Verification items for this drawing (mm, ordinates from the low corner). A direction names the side the tool comes from. Round coordinates to 2 decimals unless told otherwise and drop trailing zeros. Write each loop counter-clockwise with the first axis right and the second up, starting at its lowest first coordinate (ties: lowest second). Pieces come first, ordered by that corner, then holes. Notation, with made-up numbers: M -35,73.5 L -2,73.5 A21 ccw -2,91.5 Z; hole C 62,-39 d1. An arc over 180 degrees is marked long. One line per question, with ' | ' between items. Start each with the question number.
Q1. Tool access check on the marked faces 4 and 5. Record the directions out of +Z, -Z, +X, -X, +Y, -Y that give a thin tool (end or side, any length) a straight path to the whole face; none if there is none.
Q2. Cross-section at B-B (y = 8). Record the boundary of the cut face in (x, z).
Q3. Thickness scan on line 1 along Z through (x, y) = (18, 20.5); line 2 along Y through (x, z) = (35.5, 3.25); line 3 along Y through (x, z) = (34, 24.75). Record the ranges inside material, lowest first. Write a range as from..to.
Q4. Release check for a two-part mould opening along X. For the marked faces 1, 2 and 3 record: released by +X, released by -X, zero draft, split by the parting line, or undercut.
Q5. Cross-section at D-D (y = 20.5). Record the boundary of the cut face in (x, z), then the cut area to 3 significant figures.
Q6. Gauge pin test, flat ends, axial feed: pin 1 (6 mm diameter, centred on x = 41.5, z = 4, fed in from -Y); pin 2 (9 mm diameter, centred on x = 35.5, y = 12.5, fed in from -Z); pin 3 (7.5 mm diameter, centred on x = 22, y = 16.5, fed in from -Z); pin 4 (3 mm diameter, centred on y = 17.5, z = 7.5, fed in from -X). Record the tip position at first contact, or that the pin passes through.
Q7. Cross-section at A-A (x = 28.5). Record the boundary of the cut face in (y, z).
Q8. Cross-section at C-C (z = 23). Record the boundary of the cut face in (x, y).
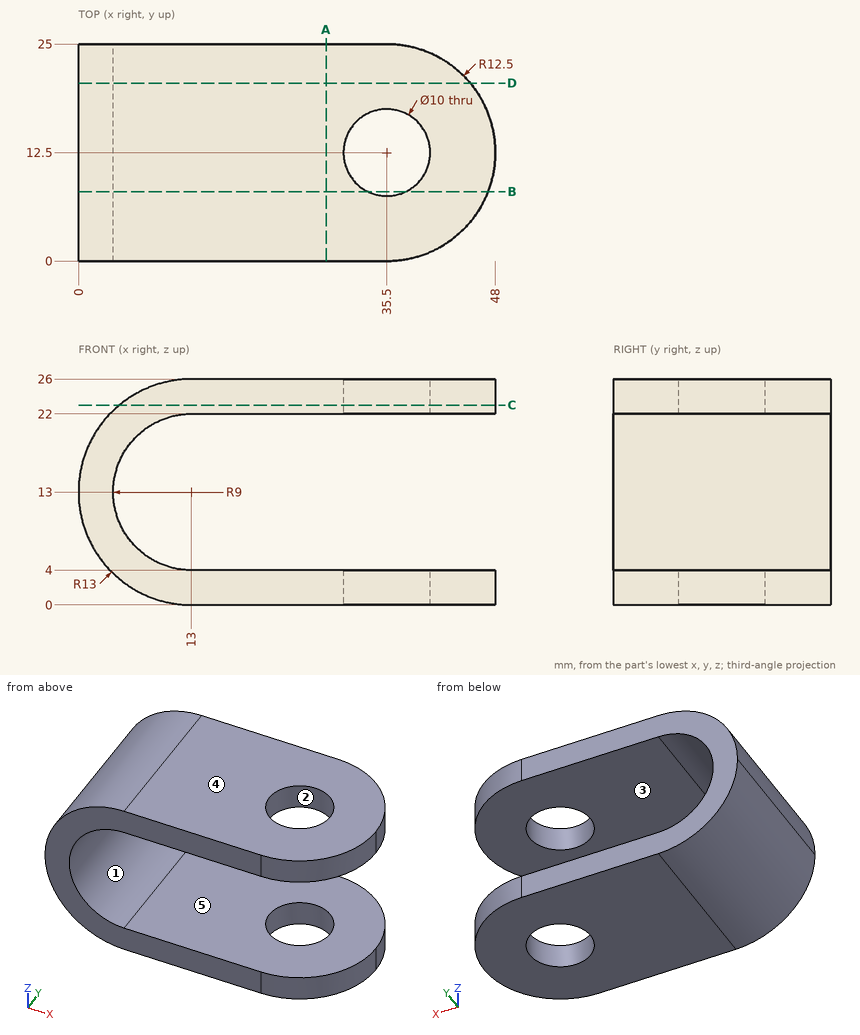
Determined:
1) face 4: +Z, +X, -X, +Y, -Y | face 5: +X, +Y, -Y
2) outline: M 13,0 L 33.32,0 L 33.32,4 L 13,4 A9 cw 13,22 L 33.32,22 L 33.32,26 L 13,26 A13 ccw Z; M 37.68,0 L 47.16,0 L 47.16,4 L 37.68,4 Z; M 37.68,22 L 47.16,22 L 47.16,26 L 37.68,26 Z
3) line 1: z = 0..4, 22..26 | line 2: y = 0..7.5, 17.5..25 | line 3: y = 0..7.73, 17.27..25
4) face 1: released by +X | face 2: undercut | face 3: zero draft
5) outline: M 13,0 L 45.1,0 L 45.1,4 L 13,4 A9 cw 13,22 L 45.1,22 L 45.1,26 L 13,26 A13 ccw Z | area: 395 mm²
6) pin 1: stops at y = 0.37 | pin 2: passes through | pin 3: stops at z = 0 | pin 4: stops at x = 0.63
7) outline: M 0,0 L 25,0 L 25,4 L 0,4 Z; M 0,22 L 25,22 L 25,26 L 0,26 Z
8) outline: M 4.69,0 L 35.5,0 A12.5 ccw 35.5,25 L 4.69,25 Z; hole C 35.5,12.5 d10
